Here's how the part is built. I have some questions about the finished solid (model axes, mm). Face numbers are marked on the shaded views. A direction names the side the tool comes from. Round coordinates to 2 decimals unless told otherwise and drop trailing zeros. Loops run counter-clockwise (first coordinate to the right, second up) from the corner with the lowest first, then second, coordinate; pieces in that order, holes last. Notation, with made-up numbers: M 54,51.5 L 109,51.5 A32 cw 109,78.5 Z; hole C 4.5,2.5 d5. An arc over 180 degrees is marked long. Answer as a JSON object with one key per item and string values.
from build123d import *

# Parameters (mm, degrees)
SKETCH_1_W          = 50
SKETCH_1_H          = 50
EXTRUDE_1_DEPTH     = 10
SKETCH_2_R          = 29
EXTRUDE_2_DEPTH     = 10
SKETCH_3_R          = 22.5
CUT_EXTRUDE_1_DEPTH = 6
SKETCH_4_R          = 34
SKETCH_4_R_2        = 29
EXTRUDE_3_DEPTH     = 23


with BuildPart() as part:
    # 草图1 → 凸台-拉伸1 (new body)
    with BuildSketch(Plane.XY):
        Rectangle(SKETCH_1_W, SKETCH_1_H)
    extrude(amount=EXTRUDE_1_DEPTH)

    # 草图2 → 凸台-拉伸2 (add)
    with BuildSketch(Plane.XZ.offset(25)):
        with BuildLine():
            Line((-25, 0), (-35.517549587, -25.142218492))
            ThreePointArc((-35.517549587, -25.142218492), (0, -78.5), (35.517549587, -25.142218492))
            Line((35.517549587, -25.142218492), (25, 0))
            Line((25, 0), (-25, 0))
        make_face()
        with Locations(Location((0, -40, 0), (0, 0, 270))):
            Circle(SKETCH_2_R, mode=Mode.SUBTRACT)
    extrude(amount=-EXTRUDE_2_DEPTH)

    # 草图3 → 切除-拉伸1 (cut)
    with BuildSketch(Plane.XY.offset(10)):
        Circle(SKETCH_3_R)
    extrude(amount=-CUT_EXTRUDE_1_DEPTH, mode=Mode.SUBTRACT)

    # 草图4 → 凸台-拉伸3 (add)
    with BuildSketch(Plane(origin=(0, -15, 0), x_dir=(1, 0, 0), z_dir=(0, 1, 0))):
        with Locations(Location((0, 40, 0), (0, 0, 90))):
            Circle(SKETCH_4_R)
        with Locations(Location((0, 40, 0), (0, 0, 90))):
            Circle(SKETCH_4_R_2, mode=Mode.SUBTRACT)
    extrude(amount=EXTRUDE_3_DEPTH)


solid = part.part
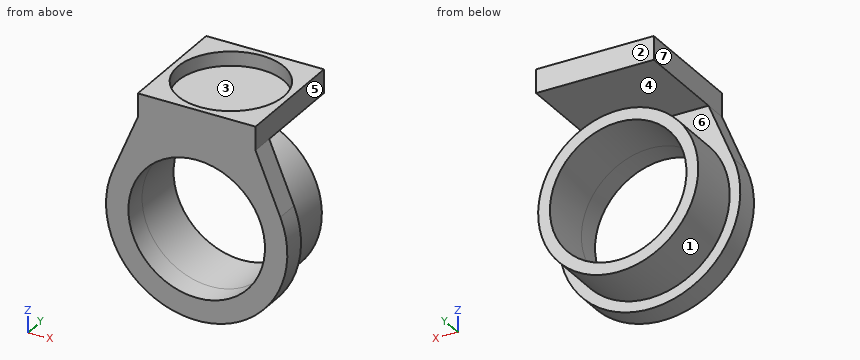
Item 1: I want a section at A-A on y = 0. List the corners of the cut face in (x, z) for me, plus the area to 3 significant figures.
Solution:
{"outline": "C 0,-40 d68; M -25,0 L 25,0 L 25,10 L 22.5,10 L 22.5,4 L -22.5,4 L -22.5,10 L -25,10 Z; hole C 0,-40 d58", "area": "1,220 mm2"}
Item 2: We'd pull the mould along Z, two halves only. Please class the marked faces 1, 2 and 3: +Z half, -Z half, draft (parallel to the pull), parting line (faces both ways), or undercut.
Solution:
{"face 1": "undercut", "face 2": "draft", "face 3": "+Z half"}
Item 3: I want a section at B-B on x = 0. List the corners of the cut face in (y, z) for me.
Solution:
{"outline": "M -25,-78.5 L -15,-78.5 L -15,-74 L 8,-74 L 8,-69 L -25,-69 Z; M -25,-11 L 8,-11 L 8,-6 L -15,-6 L -15,0 L 25,0 L 25,10 L 22.5,10 L 22.5,4 L -22.5,4 L -22.5,10 L -25,10 Z"}
Item 4: For P1, Ø10, axis at y = -4, z = -68.5, coming from the -X side; P2, Ø6, axis at x = 11.5, y = 10, coming from the -Z side; P3, Ø5, axis at y = 1, z = 3.5, coming from the -X side, each with a flat end and sliding along its axis, tell me the tip position at first contact or that it passes through.
Solution:
{"P1": "stops at x = -24.57", "P2": "stops at z = -72.71", "P3": "stops at x = -25"}
Item 5: I want a section at C-C on z = -40. List the corners of the cut face in (x, y) for me, plus the area to 3 significant figures.
Solution:
{"outline": "M -38.5,-25 L -29,-25 L -29,8 L -34,8 L -34,-15 L -38.5,-15 Z; M 29,-25 L 38.5,-25 L 38.5,-15 L 34,-15 L 34,8 L 29,8 Z", "area": "420 mm2"}
Item 6: If I drill on L1, parallel to Z at x = 1, y = 2; L2, parallel to X at y = -18.75, z = -40; L3, parallel to Z at x = 16, y = 2, over which ranges is the centre line in solid material (lowest first)? Write a range as from..to.
Solution:
{"L1": "z = -73.99..-68.98, -11.02..-6.01, 0..4", "L2": "x = -38.5..-29, 29..38.5", "L3": "z = -70..-64.19, -15.81..-10, 0..4"}
Item 7: I want a section at D-D on y = -13. List the corners of the cut face in (x, z) for me.
Solution:
{"outline": "C 0,-40 d68; M -25,0 L 25,0 L 25,10 L 18.36,10 L 18.36,4 L -18.36,4 L -18.36,10 L -25,10 Z; hole C 0,-40 d58"}
Item 8: For the marked faces 4, 5, 6 and 7, which set-ups out of +Z, -Z, +X, -X, +Y, -Y let a thin tool reach every point of the face, with its end or its side?
Solution:
{"face 4": "+X, -X, +Y", "face 5": "+Z, +X, +Y, -Y", "face 6": "+Y", "face 7": "+Z, -X, +Y, -Y"}
